```python
from build123d import *

# Parameters (mm, degrees)
F1_DEPTH = 10
F2_R     = 10
F3_R     = 30
F5_DEPTH = 10.001
F6_R     = 5
F7_DEPTH = 10.001
F9_DEPTH = 10.001


with BuildPart() as f1:
    # F0 (on Top) → F1 (new body)
    with BuildSketch(Plane.XY):
        Polygon((140, 135), (-140, 135), (-185, 60), (-185, -60), (-140, -135), (140, -135), (185, -60), (185, 60), align=None)
        Polygon((-110.982108, -86.180622), (-153.690481, -15), (-37.165167, -15), align=None, mode=Mode.SUBTRACT)
        Polygon((95.345744, -110), (-95.345744, -110), (0, -18.059461), align=None, mode=Mode.SUBTRACT)
        Polygon((37.165167, -15), (153.690481, -15), (110.982108, -86.180622), align=None, mode=Mode.SUBTRACT)
        Polygon((-153.690481, 15), (-110.982108, 86.180622), (-37.165167, 15), align=None, mode=Mode.SUBTRACT)
        Polygon((0, 18.059461), (-95.345744, 110), (95.345744, 110), align=None, mode=Mode.SUBTRACT)
        Polygon((37.165167, 15), (110.982108, 86.180622), (153.690481, 15), align=None, mode=Mode.SUBTRACT)
    extrude(amount=F1_DEPTH)

    # F2
    f2_edges = [f1.edges().sort_by_distance(p)[0] for p in [
        (-110.982108, 86.180622, 5),
        (-153.690481, 15, 5),
        (-37.165167, 15, 5),
        (153.690481, 15, 5),
        (0, 18.059461, 5),
        (-95.345744, 110, 5),
        (95.345744, 110, 5),
        (-153.690481, -15, 5),
        (-37.165167, -15, 5),
        (-110.982108, -86.180622, 5),
        (0, -18.059461, 5),
        (-95.345744, -110, 5),
        (95.345744, -110, 5),
        (153.690481, -15, 5),
        (37.165167, -15, 5),
        (110.982108, -86.180622, 5),
        (110.982108, 86.180622, 5),
        (37.165167, 15, 5),
    ]]
    fillet(f2_edges, radius=F2_R)

    # F3
    f3_edges = [f1.edges().sort_by_distance(p)[0] for p in [
        (-185, 60, 5),
        (-140, 135, 5),
        (-185, -60, 5),
        (-140, -135, 5),
        (140, -135, 5),
        (185, -60, 5),
        (185, 60, 5),
        (140, 135, 5),
    ]]
    fillet(f3_edges, radius=F3_R)

    # F4 (on face) → F5 (cut, through all)
    with BuildSketch(Plane.XY.offset(10)):
        with BuildLine():
            ThreePointArc((-170.5, -30.9), (-172.1, -32.5), (-170.5, -34.1))
            Line((-170.5, -34.1), (-165.5, -34.1))
            ThreePointArc((-165.5, -34.1), (-163.9, -32.5), (-165.5, -30.9))
            Line((-165.5, -30.9), (-170.5, -30.9))
        make_face()
        with BuildLine():
            ThreePointArc((165.5, -30.9), (163.9, -32.5), (165.5, -34.1))
            Line((165.5, -34.1), (170.5, -34.1))
            ThreePointArc((170.5, -34.1), (172.1, -32.5), (170.5, -30.9))
            Line((170.5, -30.9), (165.5, -30.9))
        make_face()
        with BuildLine():
            ThreePointArc((165.5, 34.1), (163.9, 32.5), (165.5, 30.9))
            Line((165.5, 30.9), (170.5, 30.9))
            ThreePointArc((170.5, 30.9), (172.1, 32.5), (170.5, 34.1))
            Line((170.5, 34.1), (165.5, 34.1))
        make_face()
        with BuildLine():
            ThreePointArc((-170.5, 34.1), (-172.1, 32.5), (-170.5, 30.9))
            Line((-170.5, 30.9), (-165.5, 30.9))
            ThreePointArc((-165.5, 30.9), (-163.9, 32.5), (-165.5, 34.1))
            Line((-165.5, 34.1), (-170.5, 34.1))
        make_face()
    extrude(amount=-F5_DEPTH, mode=Mode.SUBTRACT)

    # F6 (on face) → F7 (cut, through all)
    with BuildSketch(Plane.XY.offset(10)):
        with Locations((-104.5, 104.5)):
            Circle(F6_R)
        with Locations((104.5, 104.5)):
            Circle(F6_R)
        with Locations((-104.5, -104.5)):
            Circle(F6_R)
        with Locations((104.5, -104.5)):
            Circle(F6_R)
    extrude(amount=-F7_DEPTH, mode=Mode.SUBTRACT)

    # F8 (on face) → F9 (cut, through all)
    with BuildSketch(Plane.XY.offset(10)):
        with BuildLine():
            Line((-185, 25.637901), (-185, 5.637901))
            ThreePointArc((-185, 5.637901), (-178.436607, 15.637901), (-185, 25.637901))
        make_face()
        with BuildLine():
            ThreePointArc((185, 20.257118), (178.436607, 10.257118), (185, 0.257118))
            Line((185, 0.257118), (185, 20.257118))
        make_face()
    extrude(amount=-F9_DEPTH, mode=Mode.SUBTRACT)


solid = f1.part
```
Can you work these out from the model? Positions are in its coordinate system, mm. A direction names the side the tool comes from. Round coordinates to 2 decimals unless told otherwise and drop trailing zeros. Order: outer loops, then holes, each group sorted by start corner. A loop starts at its lowest first (then second) coordinate and runs counter-clockwise, first axis right, second up. Notation, with made-up numbers: (58.5, -33) -> (69.5, -33) arc R13 cw to (69.5, -24) -> close; hole circle Ø3 at (5, 42). An arc over 180 degrees is marked (long way). Return JSON: item names as keys, results as strings. Group by question number.
1. I need wall thicknesses on line 1 (Y direction, x = -45.5, z = 3); line 2 (X direction, y = 52, z = 0.5); line 3 (Y direction, x = 82, z = 5.75). Which ranges of each line are inside material? Lowest first, please. Write a range as [from, to].
2. If we section it at B-B, the plane y = 104.5: Write out the boundary of the cut face in (x, z), then the cut area to 3 significant figures.
3. We'd pull the mould along X, two halves only. Please class faces 1 (the face through (-178.44, 15.46, 5.07)), 2 (the face through (164.956, 93.407, 4.93)), 3 (the face through (-99.881, -106.415, 5.07)): released by +X, released by -X, zero draft, split by the parting line, or undercut.
4. If we section it at C-C, the plane y = -114.5: Write out the boundary of the cut face in (x, z), then the cut area to 3 significant figures.
5. Will these pins go through, and if not, where does the flat tip stop? pin 1 (5 mm diameter, centred on y = 78.5, z = 7, fed in from -X); pin 2 (1.5 mm diameter, centred on x = 167.5, z = 3, fed in from +Y); pin 3 (5.5 mm diameter, centred on x = 167.5, z = 5, fed in from -Y); pin 4 (16 mm diameter, centred on x = -104.5, y = 104.5, fed in from +Z).
6. If we section it at A-A, the plane x = -30: Write out the boundary of the cut face in (y, z), then the cut area to 3 significant figures.
7. If we section it at D-D, the plane z = 3.5: Count the separate pieces of the cut face and the enclosed holes in it, then the cut area to 3 significant figures.
8. Which directions (+Z, -Z, +X, -X, +Y, -Y) give clear straight access to the entire face, cutting with the end or side of a thin tool? Please do faces 4 (the face through (183.94, -59.59, 5.07)), 5 (the face through (-52.61, -21.41, 5.07)).
Output values:
{
 "1": {"line 1": "[-135, -110], [-61.93, 61.93], [110, 135]", "line 2": "[-185, -131.49], [-75.54, -35.2], [35.2, 75.54], [131.49, 185]", "line 3": "[-135, -58.23], [-15, 15], [58.23, 135]"},
 "2": {"outline": "(-158.3, 0) -> (-109.5, 0) -> (-109.5, 10) -> (-158.3, 10) -> close; (-99.5, 0) -> (-79.5, 0) -> (-79.5, 10) -> (-99.5, 10) -> close; (79.5, 0) -> (99.5, 0) -> (99.5, 10) -> (79.5, 10) -> close; (109.5, 0) -> (158.3, 0) -> (158.3, 10) -> (109.5, 10) -> close", "area": "1,380 mm²"},
 "3": {"face 1": "released by -X", "face 2": "released by +X", "face 3": "undercut"},
 "4": {"outline": "(-152.3, 0) -> (152.3, 0) -> (152.3, 10) -> (-152.3, 10) -> close", "area": "3,050 mm²"},
 "5": {"pin 1": "x = -175.4", "pin 2": "y = 90.42", "pin 3": "y = -93.75", "pin 4": "z = 10"},
 "6": {"outline": "(-135, 0) -> (-110, 0) -> (-110, 10) -> (-135, 10) -> close; (-46.99, 0) -> (46.99, 0) -> (46.99, 10) -> (-46.99, 10) -> close; (110, 0) -> (135, 0) -> (135, 10) -> (110, 10) -> close", "area": "1,440 mm²"},
 "7": {"separate pieces": "1", "enclosed holes": "14", "area": "59,700 mm²"},
 "8": {"face 4": "+Z, -Z, +X, -Y", "face 5": "+Z, -Z"}
}
